Geometry check sheet. Reference: the model listing, model coordinates, mm. A direction names the side the tool comes from. Give positions to 0.01 mm unless a question says otherwise; leave off trailing zeros. Write each loop counter-clockwise with the first axis right and the second up, starting at its lowest first coordinate (ties: lowest second). Pieces come first, ordered by that corner, then holes. Notation, with made-up numbers: (-16.5, -34) - (-1.5, -34) arc R38 cw to (-1.5, 5) - close; hole circle Ø11 at (-38.75, -19). An arc over 180 degrees is marked (long way). Use a Markdown table: item, result.
```python
from build123d import *

# Parameters (mm, degrees)
F0_R          = 17.3
F0_R_2        = 16.5
F1_DEPTH      = 1.3
F1_DEPTH_BACK = 1.3
F2_R          = 17.25
F3_DEPTH      = 0.5
F3_DEPTH_BACK = 0.5
F4_R          = 2.5
F5_DEPTH      = 1
F5_DEPTH_BACK = 1


with BuildPart() as f1:
    # F0 (on Top) → F1 (new body, two sides)
    with BuildSketch(Plane.XY) as f1_sk:
        Circle(F0_R)
        Circle(F0_R_2, mode=Mode.SUBTRACT)
    extrude(amount=F1_DEPTH)
    extrude(f1_sk.sketch, amount=-F1_DEPTH_BACK)

    # F2 (on Top) → F3 (join, two sides)
    with BuildSketch(Plane.XY) as f3_sk:
        Circle(F2_R)
    extrude(amount=F3_DEPTH)
    extrude(f3_sk.sketch, amount=-F3_DEPTH_BACK)

    # F4 (on Top) → F5 (cut, two sides)
    with BuildSketch(Plane.XY) as f5_sk:
        with Locations((0, 8.25)):
            Circle(F4_R)
        with Locations((-7.8462162594, 2.5493902036)):
            Circle(F4_R)
        with Locations((-4.8492283314, -6.6743902036)):
            Circle(F4_R)
        with Locations((4.8492283314, -6.6743902036)):
            Circle(F4_R)
        with Locations((7.8462162594, 2.5493902036)):
            Circle(F4_R)
    extrude(amount=-F5_DEPTH, mode=Mode.SUBTRACT)
    extrude(f5_sk.sketch, amount=F5_DEPTH_BACK, mode=Mode.SUBTRACT)


solid = f1.part
```
1) Section check A-A on x = 0. Record the boundary of the cut face in (y, z).
Working result:
| item | result |
|---|---|
| outline | (-17.3, -1.3) - (-16.5, -1.3) - (-16.5, -0.5) - (5.75, -0.5) - (5.75, 0.5) - (-16.5, 0.5) - (-16.5, 1.3) - (-17.3, 1.3) - close; (10.75, -0.5) - (16.5, -0.5) - (16.5, -1.3) - (17.3, -1.3) - (17.3, 1.3) - (16.5, 1.3) - (16.5, 0.5) - (10.75, 0.5) - close |
2) Material ranges on L1, parallel to Y at x = 0, z = -1; L2, parallel to X at y = -6.5, z = -0.1; L3, parallel to Z at x = 13.5, y = -2.5, recorded low to high. Write a range as from..to.
Working result:
| item | result |
|---|---|
| L1 | y = -17.3..-16.5, 16.5..17.3 |
| L2 | x = -16.03..-7.34, -2.36..2.36, 7.34..16.03 |
| L3 | z = -0.5..0.5 |
3) Section check B-B on y = 3. Record the boundary of the cut face in (x, z).
Working result:
| item | result |
|---|---|
| outline | (-17.04, -1.3) - (-16.22, -1.3) - (-16.22, -0.5) - (-10.31, -0.5) - (-10.31, 0.5) - (-16.22, 0.5) - (-16.22, 1.3) - (-17.04, 1.3) - close; (-5.39, -0.5) - (5.39, -0.5) - (5.39, 0.5) - (-5.39, 0.5) - close; (10.31, -0.5) - (16.22, -0.5) - (16.22, -1.3) - (17.04, -1.3) - (17.04, 1.3) - (16.22, 1.3) - (16.22, 0.5) - (10.31, 0.5) - close |
4) Set-up check for faces 1 (the flat face through (0, 0, 0.5)), 2 (the cylindrical face through (16.5, 5.2, 0)), 3 (the flat face through (0, 0, -0.5)): record each of +Z, -Z, +X, -X, +Y, -Y from which the full face is reachable in a straight line by a thin tool's end or side.
Working result:
| item | result |
|---|---|
| face 1 | +Z |
| face 2 | +Z, -Z |
| face 3 | -Z |
5) Section check C-C on x = 6. Record the boundary of the cut face in (y, z) (3 decimals).
Working result:
| item | result |
|---|---|
| outline | (-16.226, -1.3) - (-15.37, -1.3) - (-15.37, -0.5) - (-8.894, -0.5) - (-8.894, 0.5) - (-15.37, 0.5) - (-15.37, 1.3) - (-16.226, 1.3) - close; (-4.455, -0.5) - (0.864, -0.5) - (0.864, 0.5) - (-4.455, 0.5) - close; (4.235, -0.5) - (15.37, -0.5) - (15.37, -1.3) - (16.226, -1.3) - (16.226, 1.3) - (15.37, 1.3) - (15.37, 0.5) - (4.235, 0.5) - close |
6) Section check D-D on z = -0.1. Record the boundary of the cut face in (x, y).
Working result:
| item | result |
|---|---|
| outline | circle Ø34.6 at (0, 0); hole circle Ø5 at (-7.85, 2.55); hole circle Ø5 at (-4.85, -6.67); hole circle Ø5 at (0, 8.25); hole circle Ø5 at (4.85, -6.67); hole circle Ø5 at (7.85, 2.55) |
7) Depth check by flat-ended pin: P1, Ø8, axis at x = 4.85, y = -6.67, coming from the +Z side; P2, Ø1.5, axis at y = -11.5, z = 0.5, coming from the +X side. Enter the tip coordinate at first touch or a pass-through.
Working result:
| item | result |
|---|---|
| P1 | stops at z = 0.5 |
| P2 | stops at x = 13.55 |
